Geometry check sheet. Reference: the model listing, model coordinates, mm. A direction names the side the tool comes from. Round coordinates to 2 decimals unless told otherwise and drop trailing zeros. Write each loop counter-clockwise with the first axis right and the second up, starting at its lowest first coordinate (ties: lowest second). Pieces come first, ordered by that corner, then holes. Notation, with made-up numbers: (-34, -24) - (-14, -24) arc R23 ccw to (-14, 7) - close; hole circle Ø7 at (15.25, -31). An arc over 180 degrees is marked (long way). Return JSON: item names as keys, results as strings.
```python
from build123d import *

# Parameters (mm, degrees)
F0_DEPTH  = 10
F17_R     = 30
F18_DEPTH = 12
F1_R      = 24
F2_DEPTH  = 20
F3_R      = 10
F4_DEPTH  = 25
F19_R     = 10
F5_DEPTH  = 30
F6_R      = 10
F7_DEPTH  = 30
F20_R     = 16
F8_DEPTH  = 8
F21_R     = 8
F9_DEPTH  = 25
F10_R     = 10
F11_DEPTH = 35
F12_R     = 11.5
F12_R_2   = 10
F13_DEPTH = 20
F14_R     = 3.5
F15_DEPTH = 10


with BuildPart() as f0:
    # F16 (on Top) → F0 (new body)
    with BuildSketch(Plane.XY):
        with BuildLine():
            ThreePointArc((39.686269666, 45), (0, 70), (-39.686269666, 45))
            ThreePointArc((-39.686269666, 45), (-59.8699875201, -3.9477328098), (-33.4338938071, -49.8214285714))
            ThreePointArc((-33.4338938071, -49.8214285714), (0, -90), (33.4338938071, -49.8214285714))
            ThreePointArc((33.4338938071, -49.8214285714), (59.8699875201, -3.9477328098), (39.686269666, 45))
        make_face()
    extrude(amount=F0_DEPTH)

    # F17 (on Top) → F18 (join)
    with BuildSketch(Plane.XY):
        Circle(F17_R)
    extrude(amount=F18_DEPTH)

    # F1 (on face) → F2 (join)
    with BuildSketch(Plane.XY.offset(12)):
        Circle(F1_R)
    extrude(amount=F2_DEPTH)

    # F3 (on face) → F4 (cut)
    with BuildSketch(Plane.XY.offset(32)):
        Circle(F3_R)
    extrude(amount=-F4_DEPTH, mode=Mode.SUBTRACT)

    # F19 (on face) → F5 (cut)
    with BuildSketch(Plane(origin=(0, 0, 0), x_dir=(1, 0, 0), z_dir=(0, 0, -1))):
        Circle(F19_R)
    extrude(amount=-F5_DEPTH, mode=Mode.SUBTRACT)

    # F6 (on face) → F7 (cut)
    with BuildSketch(Plane.XY.offset(32)):
        Circle(F6_R)
    extrude(amount=-F7_DEPTH, mode=Mode.SUBTRACT)

    # F20 (on face) → F8 (join)
    with BuildSketch(Plane.XY.offset(10)):
        with Locations((0, -56)):
            Circle(F20_R)
    extrude(amount=F8_DEPTH)

    # F21 (on face) → F9 (cut)
    with BuildSketch(Plane.XY.offset(18)):
        with Locations((0, -56)):
            Circle(F21_R)
    extrude(amount=-F9_DEPTH, mode=Mode.SUBTRACT)

    # F10 (on face) → F11 (cut)
    with BuildSketch(Plane.XY.offset(32)):
        Circle(F10_R)
    extrude(amount=-F11_DEPTH, mode=Mode.SUBTRACT)

    # F12 (on face) → F13 (cut)
    with BuildSketch(Plane.XY.offset(32)):
        Circle(F12_R)
        Circle(F12_R_2, mode=Mode.SUBTRACT)
    extrude(amount=-F13_DEPTH, mode=Mode.SUBTRACT)

    # F14 (on face) → F15 (cut)
    with BuildSketch(Plane.XY.offset(10)):
        with Locations((-27, -56)):
            Circle(F14_R)
        with Locations((27, -56)):
            Circle(F14_R)
        with Locations((-50, 0)):
            Circle(F14_R)
        with Locations((50, 0)):
            Circle(F14_R)
        with Locations((0, 60)):
            Circle(F14_R)
    extrude(amount=-F15_DEPTH, mode=Mode.SUBTRACT)


solid = f0.part
```
(1) Section check A-A, the plane x = 0. Give the number of separate pieces and of enclosed holes in the cut face, plus the area to 3 significant figures.
Response values:
{"separate pieces": "4", "enclosed holes": "0", "area": "1,880 mm^2"}
(2) Gauge pin test, flat ends, axial feed: pin 1 (2 mm diameter, centred on x = 42, y = -1.5, fed in from +Z); pin 2 (2 mm diameter, centred on x = -47.5, z = 5, fed in from -Y); pin 3 (4 mm diameter, centred on x = 12.5, z = 9, fed in from +Y). Record the tip position at first contact, or that the pin passes through.
Response values:
{"pin 1": "stops at z = 10", "pin 2": "stops at y = -37.92", "pin 3": "stops at y = 68.73"}
(3) Access from +Z, -Z, +X, -X, +Y, -Y to the whole of each face (thin tool, end or side, straight path). Record for faces 4 (the face through (-13.5, 20.1, 12)), 5 (the face through (-1.041, -48.068, 9.126)), 6 (the face through (-3.8, -48.7, 18)).
Response values:
{"face 4": "+Z", "face 5": "+Z, -Z", "face 6": "+Z, +X, -X, -Y"}
(4) Release check for a two-part mould opening along Y. For faces 1 (the face through (-1.5, 11.4, 22.1)), 2 (the face through (10, 6, 32)), 3 (the face through (0.693, 69.995, 4.93)) record: pulls with the +Y half, pulls with the -Y half, needs draft (parallel to the pull), parting line crosses it, or undercut.
Response values:
{"face 1": "undercut", "face 2": "needs draft", "face 3": "pulls with the +Y half"}
(5) Section check C-C, the plane z = 4. Enter the section's corners in (x, y).
Response values:
{"outline": "(-39.69, 45) arc R60 ccw to (-33.43, -49.82) arc R34 ccw (long way) to (33.43, -49.82) arc R60 ccw to (39.69, 45) arc R44 ccw to start; hole circle Ø7 at (-50, 0); hole circle Ø7 at (-27, -56); hole circle Ø20 at (0, 0); hole circle Ø16 at (0, -56); hole circle Ø7 at (0, 60); hole circle Ø7 at (27, -56); hole circle Ø7 at (50, 0)"}
(6) Section check B-B, the plane y = 0. Enter the section's corners in (x, z), plus the area to 3 significant figures.
Response values:
{"outline": "(-60, 0) - (-53.5, 0) - (-53.5, 10) - (-60, 10) - close; (-46.5, 0) - (-10, 0) - (-10, 12) - (-11.5, 12) - (-11.5, 32) - (-24, 32) - (-24, 12) - (-30, 12) - (-30, 10) - (-46.5, 10) - close; (10, 0) - (46.5, 0) - (46.5, 10) - (30, 10) - (30, 12) - (24, 12) - (24, 32) - (11.5, 32) - (11.5, 12) - (10, 12) - close; (53.5, 0) - (60, 0) - (60, 10) - (53.5, 10) - close", "area": "1,440 mm^2"}
(7) Material ranges on line 1 along Y through (x, z) = (0, 14); line 2 along Y through (x, z) = (50, 3); line 3 along Y through (x, z) = (-10, 28), recorded low to high. Write a range as [from, to].
Response values:
{"line 1": "y = [-72, -64], [-48, -40], [-24, -11.5], [11.5, 24]", "line 2": "y = [-33.17, -3.5], [3.5, 33.17]", "line 3": "y = [-21.82, -5.68], [5.68, 21.82]"}
(8) Section check D-D, the plane x = -50. Enter the section's corners in (y, z).
Response values:
{"outline": "(-33.17, 0) - (-3.5, 0) - (-3.5, 10) - (-33.17, 10) - close; (3.5, 0) - (33.17, 0) - (33.17, 10) - (3.5, 10) - close"}
